Build history of the part. All positions in model axes, mm. A direction names the side the tool comes from. Round coordinates to 2 decimals unless told otherwise and drop trailing zeros. Loops run counter-clockwise (first coordinate to the right, second up) from the corner with the lowest first, then second, coordinate; pieces in that order, holes last. Notation, with made-up numbers: (2, -35.5) - (39, -35.5) arc R26 cw to (39, -15.5) - close; hole circle Ø3 at (34.5, 59.25). An arc over 180 degrees is marked (long way). Use one line per item in the form item = value. Start each with the question number.
Q1. Saw through at D-D (x = 0). Give the cut face in (y, z).
Q2. Saw through at C-C (z = 0). Give the cut face in (x, y), then the cut area to 3 significant figures.
Q3. Saw through at B-B (x = 15.5). Give the cut face in (y, z), then the cut area to 3 significant figures.
Q4. Saw through at A-A (y = 0). Give the cut face in (x, z), then the cut area to 3 significant figures.
Q5. Pin check, flat tips, straight feed: pin 1 (1.8 mm diameter, centred on y = 0, z = 0, fed in from -X); pin 2 (1.2 mm diameter, centred on x = -13.5, y = -0.5, fed in from +Z); pin 3 (0.6 mm diameter, centred on y = -0.5, z = 0, fed in from +X). Stop position of each tip, or through.
Q6. 3-axis set-ups, long thin cutter, end or side, ignore diameter. For faces 5 (the face through (10.5, 0, 2.2)), 6 (the face through (10.5, 0, -2.2)), 7 (the face through (-16, -1, 0)): which of +Z, -Z, +X, -X, +Y, -Y reach the whole face in a straight line?
Q7. Drill centre lines: line 1 (Y direction, x = 14, z = 0.05); line 2 (X direction, y = -0.7, z = -2.2); line 3 (X direction, y = -0.7, z = 0.4). Where is each one in solid material? Low to high.
Q8. Mould opens along Z. For faces 1 (the face through (12.5, 0, 0)), 2 (the face through (-10.5, 0, 2.2)), 3 (the face through (-15, 0, 1.85)), 4 (the face through (16, -1, 0)) say: released by +Z, released by -Z, zero draft, split by the parting line, or undercut.
```python
from build123d import *

# Parameters (mm, degrees)
SKETCH1_R           = 2.7
BOSS_EXTRUDE1_DEPTH = 18.5
CUT_EXTRUDE1_DEPTH  = 8
SKETCH3_R           = 1
CUT_EXTRUDE2_DEPTH  = 6


with BuildPart() as part:
    # Sketch1 → Boss-Extrude1 (new body, symmetric)
    with BuildSketch(Plane(origin=(0, 0, 0), x_dir=(0, 0, -1), z_dir=(1, 0, 0))):
        Circle(SKETCH1_R)
    extrude(amount=BOSS_EXTRUDE1_DEPTH, both=True)

    # Sketch2 → Cut-Extrude1 (cut)
    with BuildSketch(Plane(origin=(18.5, 0, 0), x_dir=(0, 0, -1), z_dir=(1, 0, 0))):
        with BuildLine():
            Line((-1.85, 1.966596044), (-1.85, -1.966596044))
            ThreePointArc((-1.85, -1.966596044), (-2.7, 0), (-1.85, 1.966596044))
        make_face()
        with BuildLine():
            Line((1.85, 1.966596044), (1.85, -1.966596044))
            ThreePointArc((1.85, -1.966596044), (2.7, 0), (1.85, 1.966596044))
        make_face()
    cut_extrude1 = extrude(amount=-CUT_EXTRUDE1_DEPTH, mode=Mode.SUBTRACT)

    # Sketch3 → Cut-Extrude2 (cut)
    with BuildSketch(Plane(origin=(18.5, 0, 0), x_dir=(0, 0, -1), z_dir=(1, 0, 0))):
        Circle(SKETCH3_R)
    cut_extrude2 = extrude(amount=-CUT_EXTRUDE2_DEPTH, mode=Mode.SUBTRACT)

    # Mirror1: Cut-Extrude1, Cut-Extrude2 across plane
    add(cut_extrude1.mirror(Plane(origin=(0, 0, 0), x_dir=(0, 0, 1), z_dir=(1, 0, 0))), mode=Mode.SUBTRACT)
    add(cut_extrude2.mirror(Plane(origin=(0, 0, 0), x_dir=(0, 0, 1), z_dir=(1, 0, 0))), mode=Mode.SUBTRACT)


solid = part.part
```
Report:
q1.outline = circle Ø5.4 at (0, 0)
q2.outline = (-18.5, -2.7) - (18.5, -2.7) - (18.5, -1) - (12.5, -1) - (12.5, 1) - (18.5, 1) - (18.5, 2.7) - (-18.5, 2.7) - (-18.5, 1) - (-12.5, 1) - (-12.5, -1) - (-18.5, -1) - close
q2.area = 176 mm²
q3.outline = (-1.97, -1.85) - (1.97, -1.85) arc R2.7 ccw to (1.97, 1.85) - (-1.97, 1.85) arc R2.7 ccw to start; hole circle Ø2 at (0, 0)
q3.area = 15.1 mm²
q4.outline = (-18.5, -1.85) - (-10.5, -1.85) - (-10.5, -2.7) - (10.5, -2.7) - (10.5, -1.85) - (18.5, -1.85) - (18.5, -1) - (12.5, -1) - (12.5, 1) - (18.5, 1) - (18.5, 1.85) - (10.5, 1.85) - (10.5, 2.7) - (-10.5, 2.7) - (-10.5, 1.85) - (-18.5, 1.85) - (-18.5, 1) - (-12.5, 1) - (-12.5, -1) - (-18.5, -1) - close
q4.area = 149 mm²
q5.pin_1 = -12.5
q5.pin_2 = 1.85
q5.pin_3 = 12.5
q6.face_5 = +Z, +X, +Y, -Y
q6.face_6 = -Z, +X, +Y, -Y
q6.face_7 = -X
q7.line_1 = -2.7 to -1, 1 to 2.7
q7.line_2 = -10.5 to 10.5
q7.line_3 = -12.5 to 12.5
q8.face_1 = undercut
q8.face_2 = zero draft
q8.face_3 = released by +Z
q8.face_4 = undercut
